Autodesk Inventor part; units mm, degrees
ref_plane "YZ Plane" through (0, 0, 0) normal (1, 0, 0) x (0, 1, 0)
ref_plane "XZ Plane" through (0, 0, 0) normal (0, 1, 0) x (-1, 0, 0)
ref_plane "XY Plane" through (0, 0, 0) normal (0, 0, 1) x (1, 0, 0)
sketch "Szkic1" plane through (0, 0, 0) normal (0, 1, 0) x (-1, 0, 0)
  circle A0 centre (0, 0) radius 6.5
  dimension "d0" = 13
extrude "Wyciągnięcie proste1" add sketch "Szkic1" along normal blind 10
sketch "Szkic2" plane through (0, 10, 0) normal (0, 1, 0) x (1, 0, 0)
  circle A0 centre (0, 0) radius 6.5
  line L0 (4, -4) -> (-4, -4)
  line L1 (-4, -4) -> (-4, 4)
  line L2 (-4, 4) -> (4, 4)
  line L3 (4, 4) -> (4, -4)
  line L4 (4, -4) -> (-4, 4) construction
  line L5 (-4, -4) -> (4, 4) construction
  dimension "d3" = 8
  dimension "d4" = 8
extrude "Wyciągnięcie proste2" cut sketch "Szkic2" against normal blind 3.5 contours L0 L1 L2 L3
chamfer "Faza1" distance 0.5 angle 45 4 edges at (-4, 10, 0) (0, 10, 4) (4, 10, 0) (0, 10, -4)
chamfer "Faza2" distance 0.5 angle 45 1 edges at (6.5, 0, 0)
properties part number "koncowka z miejscem na magnes neodymowy 7x7x3"
Input: part model. Units: mm. Frame: model coordinates. A direction names the side the tool comes from. Give positions to 0.01 mm unless a question says otherwise; leave off trailing zeros. Order: outer loops, then holes, each group sorted by start corner. A loop starts at its lowest first (then second) coordinate and runs counter-clockwise, first axis right, second up.
1. Section D-D on y = 1. Return the cut outline in (x, z), and give its area (3 significant figures).
Derived:
outline: circle Ø13 at (0, 0)
area: 133 mm2
2. Material intervals for L1, parallel to X at y = 6.75, z = -3; L2, parallel to Y at x = 1.75, z = 2.75; L3, parallel to Z at x = -1, y = 7.25, sorted ascending.
Derived:
L1: x = -5.77 to -4, 4 to 5.77
L2: y = 0 to 6.5
L3: z = -6.42 to -4, 4 to 6.42
3. Reachability of faces 1 (the flat face through (0, 6.5, 0)), 2 (the flat face through (0, 0, 0)) from +Z, -Z, +X, -X, +Y, -Y: full face, straight path, thin tool, end or side. Return the list, or none.
Derived:
face 1: +Y
face 2: +Z, -Z, +X, -X, -Y
4. Section B-B on z = 0. Return the cut outline in (x, y), and give its area (4 significant figures).
Derived:
outline: (-6.5, 0.5) - (-6, 0) - (6, 0) - (6.5, 0.5) - (6.5, 10) - (4.5, 10) - (4, 9.5) - (4, 6.5) - (-4, 6.5) - (-4, 9.5) - (-4.5, 10) - (-6.5, 10) - close
area: 101.5 mm2
5. Section C-C on y = 7.5. Return the cut outline in (x, z).
Derived:
outline: circle Ø13 at (0, 0); hole (-4, -4) - (4, -4) - (4, 4) - (-4, 4) - close
6. Section A-A on x = 0. Return the cut outline in (y, z), and give its area (4 significant figures).
Derived:
outline: (0, -6) - (0.5, -6.5) - (10, -6.5) - (10, -4.5) - (9.5, -4) - (6.5, -4) - (6.5, 4) - (9.5, 4) - (10, 4.5) - (10, 6.5) - (0.5, 6.5) - (0, 6) - close
area: 101.5 mm2
7. Mould query, pull axis Z, two halves, no side actions, for faces 3 (the flat face through (0, 10, -5)), 4 (the cylindrical face through (5.158, 5.184, 3.955)), 5 (the flat face through (4, 8, 0)). Classes: released by +Z, released by -Z, zero draft, split by the parting line, or undercut.
Derived:
face 3: zero draft
face 4: split by the parting line
face 5: undercut
8. Pin query (flat end, axial travel): pin 1 (5 mm diameter, centred on y = 6.5, z = -1, fed in from -X); pin 2 (4 mm diameter, centred on x = 3.5, y = 1.5, fed in from -Z); pin 3 (2.5 mm diameter, centred on x = -1.5, y = 8, fed in from +Z); pin 4 (2.5 mm diameter, centred on y = 8.5, z = 2, fed in from +X). Return the tip coordinate at first contact, or that it passes through.
Derived:
pin 1: stops at x = -6.5
pin 2: stops at z = -6.32
pin 3: stops at z = 6.5
pin 4: stops at x = 6.46
